Source: CAD feature listing. Evaluate the final solid. Frame: model axes, mm. Face numbers are marked on the shaded views. Round coordinates to 2 decimals unless told otherwise and drop trailing zeros. Order: outer loops, then holes, each group sorted by start corner. A loop starts at its lowest first (then second) coordinate and runs counter-clockwise, first axis right, second up. Notation, with made-up numbers: (73.5, -1.75) -> (99.5, -1.75) arc R34 ccw to (99.5, 33.25) -> close; hole circle Ø3 at (7, 75). An arc over 180 degrees is marked (long way). Answer as CSV lines item,"result". Start each with the question number.
(1) Section query B-B (y = -8.5). Output: boundary loops of the cut face in (x, z).
(2) Contact query for flat-ended pins moving along their axis: P1, Ø1.5, axis at y = -8, z = 9.5, coming from the -X side; P2, Ø2.5, axis at y = -8.5, z = 22, coming from the +X side; P3, Ø1.5, axis at x = 0, y = 0, coming from the -Z side; P4, Ø3, axis at x = -5.5, z = 13.5, coming from the -Y side. Output: stop coordinate, or through.
(3) Section query A-A (z = 8.5). Output: boundary loops of the cut face in (x, y).
(4) Line query: line 1 along Y through (x, z) = (0, 26.75); line 2 along X through (y, z) = (0, 24); line 3 along Y through (x, z) = (-2.25, 19.25). Output: solid intervals per line, ascending. Write a range as from..to.
(5) Pull-direction query (X, two-part tool) for the marked faces 1, 2 and 3; classes: +X half, -X half, draft (parallel to the pull), parting line (faces both ways), or undercut.
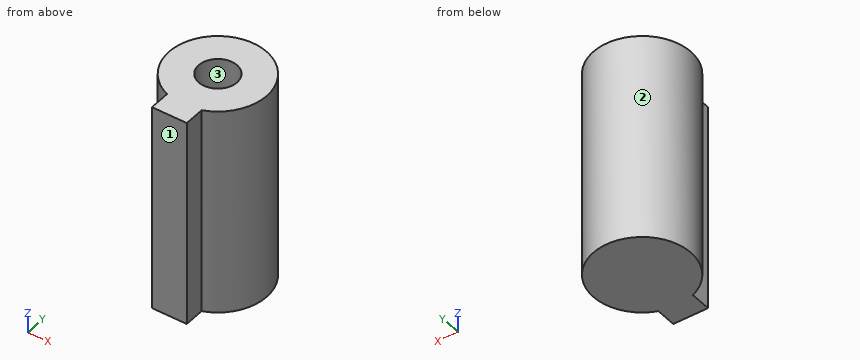
```python
from build123d import *

# Parameters (mm, degrees)
F1_DEPTH = 30
F3_D     = 5.5
F3_DEPTH = 12
F3_TIP   = 1.6523667023


with BuildPart() as f1:
    # F0 (on Top) → F1 (new body)
    with BuildSketch(Plane.XY):
        with BuildLine():
            Line((2.4379568888, -9.5), (2.4379568888, -6.5617349999))
            ThreePointArc((2.4379568888, -6.5617349999), (0.0664242114, 6.9996848375), (-2.5620431112, -6.5142869983))
            Line((-2.5620431112, -6.5142869983), (-2.5620431112, -9.5))
            Line((-2.5620431112, -9.5), (2.4379568888, -9.5))
        make_face()
    extrude(amount=F1_DEPTH)

    # F3
    with Locations(Plane.XY.offset(30)):
        with Locations((0, 0)):
            Hole(F3_D / 2, depth=F3_DEPTH)
            with Locations((0, 0, -(F3_DEPTH + F3_TIP / 2))):  # 118° drill point
                Cone(0, F3_D / 2, F3_TIP, mode=Mode.SUBTRACT)


solid = f1.part
```
Answer block:
1,outline,"(-2.56, 0) -> (2.44, 0) -> (2.44, 30) -> (-2.56, 30) -> close"
2,P1,"x = -2.56"
2,P2,"x = 2.44"
2,P3,"z = 0"
2,P4,"y = -5.74"
3,outline,"(-2.56, -9.5) -> (2.44, -9.5) -> (2.44, -6.56) arc R7 ccw (long way) to (-2.56, -6.51) -> close"
4,line 1,"-9.5..-2.75, 2.75..7"
4,line 2,"-7..-2.75, 2.75..7"
4,line 3,"-9.5..-1.58, 1.58..6.63"
5,face 1,"draft"
5,face 2,"parting line"
5,face 3,"undercut"
